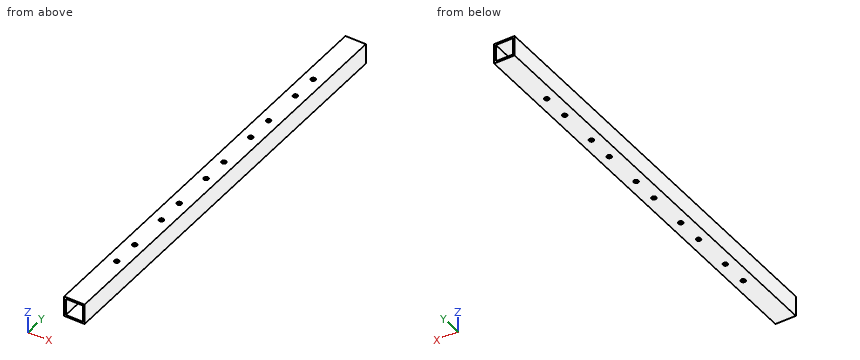
from build123d import *

# Parameters (mm, degrees)
F0_W       = 19.05
F0_H       = 19.05
F0_W_2     = 15.875
F0_H_2     = 15.875
F1_DEPTH   = 200.025
F2_R       = 2.15265
F1_FACE1_W = 19.05
F1_FACE1_H = 400.05
F3_DEPTH   = 25.4


with BuildPart() as f1:
    # F0 (on Front) → F1 (new body, symmetric)
    with BuildSketch(Plane.XZ):
        Rectangle(F0_W, F0_H)
        Rectangle(F0_W_2, F0_H_2, mode=Mode.SUBTRACT)
    extrude(amount=F1_DEPTH, both=True)

    # F2 (on face) + F1_face1 (on face) → F3 (cut)
    with BuildSketch(Plane.XY.offset(9.525)):
        with Locations((0, 12.7)):
            Circle(F2_R)
        with Locations((0, -12.7)):
            Circle(F2_R)
        with Locations((0, 76.2)):
            Circle(F2_R)
        with Locations((0, 50.8)):
            Circle(F2_R)
        with Locations((0, 139.7)):
            Circle(F2_R)
        with Locations((0, 114.3)):
            Circle(F2_R)
        with Locations((0, -50.8)):
            Circle(F2_R)
        with Locations((0, -76.2)):
            Circle(F2_R)
        with Locations((0, -114.3)):
            Circle(F2_R)
        with Locations((0, -139.7)):
            Circle(F2_R)
    with BuildSketch(Plane(origin=(0, 0, -9.525), x_dir=(1, 0, 0), z_dir=(0, 0, -1))):
        Rectangle(F1_FACE1_W, F1_FACE1_H)
    extrude(amount=-F3_DEPTH, dir=(0, 0, 1), mode=Mode.SUBTRACT)


solid = f1.part
The model under review builds one solid part; all positions refer to its coordinate system, in mm. Give positions to 0.01 mm unless a question says otherwise; leave off trailing zeros. Write each loop counter-clockwise with the first axis right and the second up, starting at its lowest first coordinate (ties: lowest second). Pieces come first, ordered by that corner, then holes. Notation, with made-up numbers: M 16.5,-10.75 L 45.5,-10.75 A18 ccw 45.5,-1.75 Z; hole C -8,22.25 d11. An arc over 180 degrees is marked long. One line per question, with ' | ' between items. Start each with the question number.
Item 1: We need section A-A on y = -125.5. Write out the cut boundary in (x, z) (1 decimal), plus the area to 3 significant figures.
Item 2: Wall thickness on line 1 (Z direction, x = 5.25, y = 165.5) (1 decimal): over which ranges is the line inside the solid? List them lowest first. Write a range as from..to.
Item 3: We need section B-B on z = 4.25. Write out the cut boundary in (x, y) (1 decimal), plus the area to 3 significant figures.
Results found:
1) outline: M -9.5,-9.5 L 9.5,-9.5 L 9.5,9.5 L -9.5,9.5 Z; hole M -7.9,-7.9 L 7.9,-7.9 L 7.9,7.9 L -7.9,7.9 Z | area: 111 mm2
2) line 1: z = -9.5..-7.9, 7.9..9.5
3) outline: M -9.5,-200 L -7.9,-200 L -7.9,200 L -9.5,200 Z; M 7.9,-200 L 9.5,-200 L 9.5,200 L 7.9,200 Z | area: 1,270 mm2
